Build history of the part. All positions in model axes, mm. Coordinates: 2 decimals unless noted, no trailing zeros. Loops run counter-clockwise (first coordinate to the right, second up) from the corner with the lowest first, then second, coordinate; pieces in that order, holes last.
Item 1: Cut at B-B (x = -90). List the corners of the cut face in (y, z).
Item 2: Cut at D-D (x = 60.5). List the corners of the cut face in (y, z).
Item 3: Cut at C-C (z = 7). Count the separate pieces of the cut face and the enclosed holes in it, and give its area (3 significant figures).
Item 4: Cut at A-A (y = 17.5). List the corners of the cut face in (x, z).
Item 5: Drill centre lines: line 1 along Y through (x, z) = (-90, 3.75); line 2 along X through (y, z) = (15.5, 4); line 3 along X through (y, z) = (21, 3.5). Where is each one in solid material? Low to high.
Item 6: Mould opens along X. For faces 1 (the face through (105, 0, 5)), 2 (the face through (-1, 0, 0)), 3 (the face through (-94.496, 17.698, 5.07)), 4 (the face through (-94.496, -12.302, 5.07)) say: released by +X, released by -X, zero draft, split by the parting line, or undercut.
Item 7: Flat gauge pins, fed straight in: pin 1 (5.5 mm diameter, centred on x = 90, y = -12.5, fed in from +Z); pin 2 (1.5 mm diameter, centred on x = -21.5, y = -11, fed in from -Z). Where does each tip first touch, or does it go through?
from build123d import *

# Parameters (mm, degrees)
SKETCH1_W           = 210
SKETCH1_H           = 65
BOSS_EXTRUDE1_DEPTH = 10
CUT_EXTRUDE1_REACH  = 112.369
SKETCH2_R           = 4.5


with BuildPart() as part:
    # Sketch1 → Boss-Extrude1 (new body)
    with BuildSketch(Plane.XY):
        Rectangle(SKETCH1_W, SKETCH1_H)
    extrude(amount=BOSS_EXTRUDE1_DEPTH)

    # Sketch2 → Cut-Extrude1 (cut, up to next)
    with BuildSketch(Plane.XY.offset(10), mode=Mode.PRIVATE) as cut_extrude1_sk1:
        with Locations((-90, -12.5)):
            Circle(SKETCH2_R)
    cut_extrude1_tool1 = extrude(cut_extrude1_sk1.sketch, amount=-CUT_EXTRUDE1_REACH, mode=Mode.PRIVATE) & part.part
    # Sketch2 → Cut-Extrude1 (cut, up to next)
    with BuildSketch(Plane.XY.offset(10), mode=Mode.PRIVATE) as cut_extrude1_sk2:
        with Locations((-90, 17.5)):
            Circle(SKETCH2_R)
    cut_extrude1_tool2 = extrude(cut_extrude1_sk2.sketch, amount=-CUT_EXTRUDE1_REACH, mode=Mode.PRIVATE) & part.part
    # Sketch2 → Cut-Extrude1 (cut, up to next)
    with BuildSketch(Plane.XY.offset(10), mode=Mode.PRIVATE) as cut_extrude1_sk3:
        with Locations((-60, 17.5)):
            Circle(SKETCH2_R)
    cut_extrude1_tool3 = extrude(cut_extrude1_sk3.sketch, amount=-CUT_EXTRUDE1_REACH, mode=Mode.PRIVATE) & part.part
    # Sketch2 → Cut-Extrude1 (cut, up to next)
    with BuildSketch(Plane.XY.offset(10), mode=Mode.PRIVATE) as cut_extrude1_sk4:
        with Locations((-60, -12.5)):
            Circle(SKETCH2_R)
    cut_extrude1_tool4 = extrude(cut_extrude1_sk4.sketch, amount=-CUT_EXTRUDE1_REACH, mode=Mode.PRIVATE) & part.part
    # Sketch2 → Cut-Extrude1 (cut, up to next)
    with BuildSketch(Plane.XY.offset(10), mode=Mode.PRIVATE) as cut_extrude1_sk5:
        with Locations((60, 17.5)):
            Circle(SKETCH2_R)
    cut_extrude1_tool5 = extrude(cut_extrude1_sk5.sketch, amount=-CUT_EXTRUDE1_REACH, mode=Mode.PRIVATE) & part.part
    # Sketch2 → Cut-Extrude1 (cut, up to next)
    with BuildSketch(Plane.XY.offset(10), mode=Mode.PRIVATE) as cut_extrude1_sk6:
        with Locations((90, 17.5)):
            Circle(SKETCH2_R)
    cut_extrude1_tool6 = extrude(cut_extrude1_sk6.sketch, amount=-CUT_EXTRUDE1_REACH, mode=Mode.PRIVATE) & part.part
    # Sketch2 → Cut-Extrude1 (cut, up to next)
    with BuildSketch(Plane.XY.offset(10), mode=Mode.PRIVATE) as cut_extrude1_sk7:
        with Locations((60, -12.5)):
            Circle(SKETCH2_R)
    cut_extrude1_tool7 = extrude(cut_extrude1_sk7.sketch, amount=-CUT_EXTRUDE1_REACH, mode=Mode.PRIVATE) & part.part
    # Sketch2 → Cut-Extrude1 (cut, up to next)
    with BuildSketch(Plane.XY.offset(10), mode=Mode.PRIVATE) as cut_extrude1_sk8:
        with Locations((90, -12.5)):
            Circle(SKETCH2_R)
    cut_extrude1_tool8 = extrude(cut_extrude1_sk8.sketch, amount=-CUT_EXTRUDE1_REACH, mode=Mode.PRIVATE) & part.part
    add(cut_extrude1_tool1.solids().sort_by_distance((-90, -12.5, 10))[0], mode=Mode.SUBTRACT)
    add(cut_extrude1_tool2.solids().sort_by_distance((-90, 17.5, 10))[0], mode=Mode.SUBTRACT)
    add(cut_extrude1_tool3.solids().sort_by_distance((-60, 17.5, 10))[0], mode=Mode.SUBTRACT)
    add(cut_extrude1_tool4.solids().sort_by_distance((-60, -12.5, 10))[0], mode=Mode.SUBTRACT)
    add(cut_extrude1_tool5.solids().sort_by_distance((60, 17.5, 10))[0], mode=Mode.SUBTRACT)
    add(cut_extrude1_tool6.solids().sort_by_distance((90, 17.5, 10))[0], mode=Mode.SUBTRACT)
    add(cut_extrude1_tool7.solids().sort_by_distance((60, -12.5, 10))[0], mode=Mode.SUBTRACT)
    add(cut_extrude1_tool8.solids().sort_by_distance((90, -12.5, 10))[0], mode=Mode.SUBTRACT)


solid = part.part
Filled sheet:
1. outline: (-32.5, 0) - (-17, 0) - (-17, 10) - (-32.5, 10) - close; (-8, 0) - (13, 0) - (13, 10) - (-8, 10) - close; (22, 0) - (32.5, 0) - (32.5, 10) - (22, 10) - close
2. outline: (-32.5, 0) - (-16.97, 0) - (-16.97, 10) - (-32.5, 10) - close; (-8.03, 0) - (13.03, 0) - (13.03, 10) - (-8.03, 10) - close; (21.97, 0) - (32.5, 0) - (32.5, 10) - (21.97, 10) - close
3. separate pieces: 1
3. enclosed holes: 8
3. area: 13,100 mm2
4. outline: (-105, 0) - (-94.5, 0) - (-94.5, 10) - (-105, 10) - close; (-85.5, 0) - (-64.5, 0) - (-64.5, 10) - (-85.5, 10) - close; (-55.5, 0) - (55.5, 0) - (55.5, 10) - (-55.5, 10) - close; (64.5, 0) - (85.5, 0) - (85.5, 10) - (64.5, 10) - close; (94.5, 0) - (105, 0) - (105, 10) - (94.5, 10) - close
5. line 1: y = -32.5 to -17, -8 to 13, 22 to 32.5
5. line 2: x = -105 to -94.03, -85.97 to -64.03, -55.97 to 55.97, 64.03 to 85.97, 94.03 to 105
5. line 3: x = -105 to -92.83, -87.17 to -62.83, -57.17 to 57.17, 62.83 to 87.17, 92.83 to 105
6. face 1: released by +X
6. face 2: zero draft
6. face 3: undercut
6. face 4: undercut
7. pin 1: passes through
7. pin 2: stops at z = 0
